Read the model definition and answer for the solid it produces. Units are mm, in the model's axes. Face numbers are marked on the shaded views. A direction names the side the tool comes from. Round coordinates to 2 decimals unless told otherwise and drop trailing zeros. Write each loop counter-clockwise with the first axis right and the second up, starting at its lowest first coordinate (ties: lowest second). Pieces come first, ordered by that corner, then holes. Notation, with made-up numbers: M 38,83.25 L 48,83.25 A14 ccw 48,109.25 Z; hole C 2,7.5 d10. An arc over 180 degrees is marked long. Use one line per item in the form item = value. Start each with the question number.
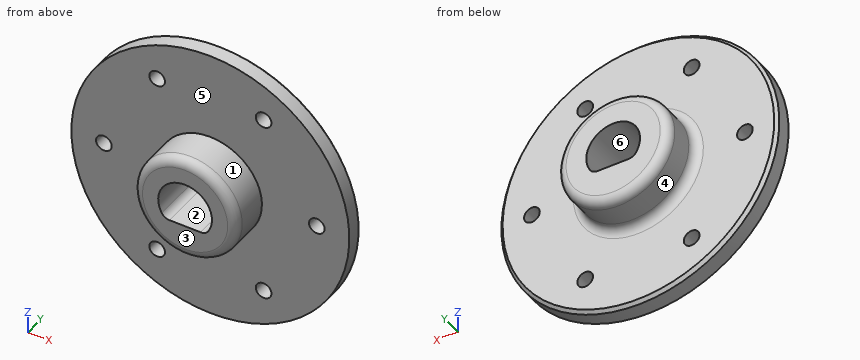
```python
from build123d import *

# Parameters (mm, degrees)
SKETCH1_R           = 31
SKETCH1_R_2         = 1.75
BOSS_EXTRUDE1_DEPTH = 4
SKETCH2_R           = 12.5
BOSS_EXTRUDE2_DEPTH = 9
FILLET2_R           = 2
CHAMFER2_SIZE       = 0.7
SKETCH6_R           = 11.5
BOSS_EXTRUDE3_DEPTH = 9
FILLET3_R           = 2
CUT_EXTRUDE3_DEPTH  = 50.050993874
FILLET4_R           = 2


with BuildPart() as part:
    # Sketch1 → Boss-Extrude1 (new body)
    with BuildSketch(Plane(origin=(0, 0, 0), x_dir=(1, 0, 0), z_dir=(0, 1, 0))):
        with Locations(Location((0, 0, 0), (0, 0, 270))):
            Circle(SKETCH1_R)
        with Locations(Location((-11.875, 20.56810334, 0), (0, 0, 270))):
            Circle(SKETCH1_R_2, mode=Mode.SUBTRACT)
        with Locations(Location((11.875, 20.56810334, 0), (0, 0, 270))):
            Circle(SKETCH1_R_2, mode=Mode.SUBTRACT)
        with Locations(Location((23.75, 0, 0), (0, 0, 270))):
            Circle(SKETCH1_R_2, mode=Mode.SUBTRACT)
        with Locations(Location((11.875, -20.56810334, 0), (0, 0, 270))):
            Circle(SKETCH1_R_2, mode=Mode.SUBTRACT)
        with Locations(Location((-11.875, -20.56810334, 0), (0, 0, 270))):
            Circle(SKETCH1_R_2, mode=Mode.SUBTRACT)
        with Locations(Location((-23.75, 0, 0), (0, 0, 270))):
            Circle(SKETCH1_R_2, mode=Mode.SUBTRACT)
    extrude(amount=BOSS_EXTRUDE1_DEPTH)

    # Sketch2 → Boss-Extrude2 (add)
    with BuildSketch(Plane(origin=(0, 4, 0), x_dir=(1, 0, 0), z_dir=(0, 1, 0))):
        with Locations(Location((0, 0, 0), (0, 0, 270))):
            Circle(SKETCH2_R)
    extrude(amount=BOSS_EXTRUDE2_DEPTH)

    # Fillet2
    fillet2_edges = [part.edges().sort_by_distance(p)[0] for p in [
        (0, 4, -12.5),
        (0, 13, -12.5),
    ]]
    fillet(fillet2_edges, radius=FILLET2_R)

    # Chamfer2
    chamfer2_edges = [part.edges().sort_by_distance(p)[0] for p in [
        (0, 4, -31),
    ]]
    chamfer(chamfer2_edges, length=CHAMFER2_SIZE)

    # Sketch6 → Boss-Extrude3 (add)
    with BuildSketch(Plane(origin=(0, 0, 0), x_dir=(-1, 0, 0), z_dir=(0, -1, 0))):
        with Locations(Location((0, 0, 0), (0, 0, 270))):
            Circle(SKETCH6_R)
    extrude(amount=BOSS_EXTRUDE3_DEPTH)

    # Fillet3
    fillet3_edges = [part.edges().sort_by_distance(p)[0] for p in [
        (0, -9, -11.5),
    ]]
    fillet(fillet3_edges, radius=FILLET3_R)

    # Sketch7 → Cut-Extrude3 (cut, through all)
    with BuildSketch(Plane(origin=(0, -9, 0), x_dir=(-1, 0, 0), z_dir=(0, -1, 0))):
        with BuildLine():
            Line((4.472135955, 4), (-4.472135955, 4))
            ThreePointArc((-4.472135955, 4), (0, -6), (4.472135955, 4))
        make_face()
    extrude(amount=-CUT_EXTRUDE3_DEPTH, mode=Mode.SUBTRACT)

    # Fillet4
    fillet4_edges = [part.edges().sort_by_distance(p)[0] for p in [
        (-4.472135955, 2, -4),
        (4.472135955, 2, -4),
    ]]
    fillet(fillet4_edges, radius=FILLET4_R)


solid = part.part
```
Q1. A tool of negligible diameter and unlimited length cuts with its end or side. For the marked faces 4, 5 and 6, from which of +Z, -Z, +X, -X, +Y, -Y can it reach the whole face along a straight path? Write none if from no direction.
Q2. For a pull along Z with two mould halves and no side action, classify the marked faces 1, 2 and 3 as +Z half, -Z half, draft (parallel to the pull), parting line (faces both ways), or undercut.
Q3. Find section A-A on z = 0. Count the separate pieces of the cut face and the enclosed holes in it, and give its area (3 significant figures).
Q4. Find section C-C on y = -1.5. Write down the section's boundary in (x, z).
Q5. Find section B-B on y = 8.5. Write down the section's boundary in (x, z).
Q6. Each of these flat-tipped pins is pushed along its axis until it touches: pin 1 Ø2 at (y, z) = (4, -1.5) entering from +X; pin 2 Ø4.5 at (x, z) = (11.88, 20.57) entering from -Y; pin 3 Ø1.5 at (x, z) = (-15.5, -23.5) entering from +Y. Where does it stop, or does it pass through?
Q7. Straight lines are drawn through the part: line 1 (X direction, y = 8.75, z = 0); line 2 (Z direction, x = 11, y = 3); line 3 (Y direction, x = -18, z = -14.5). For each, find the intervals that lie inside material, in ascending order. Write a range as [from, to].
Response:
q1.face_4 = +Y
q1.face_5 = -Y
q1.face_6 = +Y, -Y
q2.face_1 = parting line
q2.face_2 = undercut
q2.face_3 = draft
q3.separate_pieces = 4
q3.enclosed_holes = 0
q3.area = 386 mm²
q4.outline = C 0,0 d23; hole M -5.2,-3 A2 ccw -3.46,-4 L 3.46,-4 A2 ccw 5.2,-3 A6 ccw long Z
q5.outline = C 0,0 d25; hole M -5.2,-3 A2 ccw -3.46,-4 L 3.46,-4 A2 ccw 5.2,-3 A6 ccw long Z
q6.pin_1 = 30.99
q6.pin_2 = 0
q6.pin_3 = 4
q7.line_1 = [-12.5, -6], [6, 12.5]
q7.line_2 = [-28.98, -22.08], [-19.05, 19.05], [22.08, 28.98]
q7.line_3 = [0, 4]
